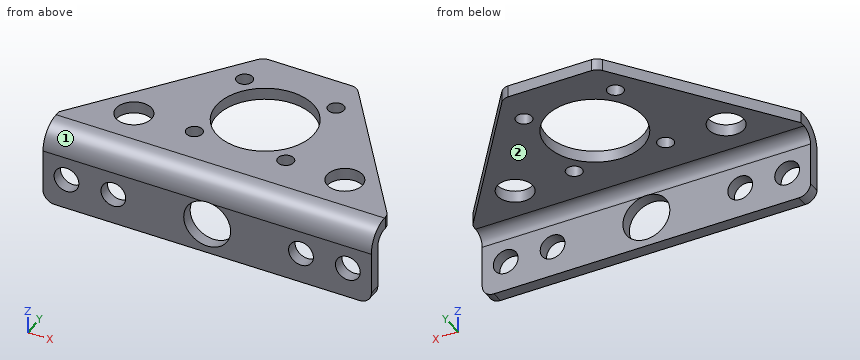
from build123d import *

# Parameters (mm, degrees)
BOSS_EXTRUDE1_DEPTH = 44.45
SKETCH2_OUTSIDE_W   = 111.802
SKETCH2_OUTSIDE_H   = 43.857
SKETCH2_OUTSIDE_R   = 3.3528
SKETCH2_OUTSIDE_R_2 = 6.35
CUT_EXTRUDE3_DEPTH  = 51.8
SKETCH3_OUTSIDE_W   = 111.802
SKETCH3_OUTSIDE_H   = 73.702
SKETCH3_OUTSIDE_R   = 2.1463
SKETCH3_OUTSIDE_R_2 = 13.0556
SKETCH3_OUTSIDE_R_3 = 4.7625
SKETCH3_OUTSIDE_R_4 = 4.743651166
CUT_EXTRUDE4_DEPTH  = 21.948744152


with BuildPart() as part:
    # Sketch1 → Boss-Extrude1 (new body, symmetric)
    with BuildSketch(Plane.ZY):
        with BuildLine():
            Line((-20.955, -28.575), (-6.5, -28.575))
            ThreePointArc((-6.5, -28.575), (-1.903805922, -26.671194078), (0, -22.075))
            Line((0, -22.075), (0, 22.225))
            Line((0, 22.225), (-3.175, 22.225))
            Line((-3.175, 22.225), (-3.175, -22.15))
            ThreePointArc((-3.175, -22.15), (-4.126902961, -24.448097039), (-6.425, -25.4))
            Line((-6.425, -25.4), (-20.955, -25.4))
            Line((-20.955, -25.4), (-20.955, -28.575))
        make_face()
    extrude(amount=BOSS_EXTRUDE1_DEPTH, both=True)

    # Sketch2 outside → Cut-Extrude3 (cut, through all)
    with BuildSketch(Plane.XZ.offset(28.575)):
        with Locations((0, -10.4775)):
            Rectangle(SKETCH2_OUTSIDE_W, SKETCH2_OUTSIDE_H)
        with BuildLine():
            Line((-41.280304188, -20.948744152), (41.275, -20.948744152))
            ThreePointArc((41.275, -20.948744152), (43.52006403, -20.018808183), (44.45, -17.773744152))
            Line((44.45, -17.773744152), (44.45, 4.535349672))
            Line((44.45, 4.535349672), (-44.455304188, 4.535349672))
            Line((-44.455304188, 4.535349672), (-44.455304188, -17.773744152))
            ThreePointArc((-44.455304188, -17.773744152), (-43.525368218, -20.018808183), (-41.280304188, -20.948744152))
        make_face(mode=Mode.SUBTRACT)
        with Locations((-38.1, -12.7)):
            Circle(SKETCH2_OUTSIDE_R)
        with Locations((-25.4, -12.7)):
            Circle(SKETCH2_OUTSIDE_R)
        with Locations((0, -12.7)):
            Circle(SKETCH2_OUTSIDE_R_2)
        with Locations((25.4, -12.7)):
            Circle(SKETCH2_OUTSIDE_R)
        with Locations((38.1, -12.7)):
            Circle(SKETCH2_OUTSIDE_R)
    extrude(amount=-CUT_EXTRUDE3_DEPTH, mode=Mode.SUBTRACT)

    # Sketch3 outside → Cut-Extrude4 (cut, through all)
    with BuildSketch(Plane.XY):
        with Locations((0, -3.175)):
            Rectangle(SKETCH3_OUTSIDE_W, SKETCH3_OUTSIDE_H)
        with BuildLine():
            Line((-13.653876698, 20.947210396), (-44.450826739, -20.631729198))
            Line((-44.450826739, -20.631729198), (-44.450826739, -28.575))
            Line((-44.450826739, -28.575), (44.45, -28.575))
            Line((44.45, -28.575), (44.45, -21.674369393))
            ThreePointArc((44.45, -21.674369393), (44.29004015, -20.679302615), (43.826278492, -19.784500865))
            Line((43.826278492, -19.784500865), (13.654037866, 20.947321174))
            ThreePointArc((13.654037866, 20.947321174), (12.531096243, 21.893026448), (11.102759374, 22.232452646))
            Line((11.102759374, 22.232452646), (-11.10251615, 22.232452646))
            ThreePointArc((-11.10251615, 22.232452646), (-12.530914579, 21.892995438), (-13.653876698, 20.947210396))
        make_face(mode=Mode.SUBTRACT)
        with Locations((-12.374792935, 12.374792935)):
            Circle(SKETCH3_OUTSIDE_R)
        with Locations((12.374792935, 12.374792935)):
            Circle(SKETCH3_OUTSIDE_R)
        Circle(SKETCH3_OUTSIDE_R_2)
        with Locations((-28.575, -12.7)):
            Circle(SKETCH3_OUTSIDE_R_3)
        with Locations((-12.374792935, -12.374792935)):
            Circle(SKETCH3_OUTSIDE_R)
        with Locations((12.374792935, -12.374792935)):
            Circle(SKETCH3_OUTSIDE_R)
        with Locations((28.564780042, -12.715837646)):
            Circle(SKETCH3_OUTSIDE_R_4)
    extrude(amount=-CUT_EXTRUDE4_DEPTH, mode=Mode.SUBTRACT)


solid = part.part
Check sheet for the modelled part. Datum: model origin and axes. Units: mm. Face numbers are marked on the shaded views. A direction names the side the tool comes from. Give positions to 0.01 mm unless a question says otherwise; leave off trailing zeros. Order: outer loops, then holes, each group sorted by start corner. A loop starts at its lowest first (then second) coordinate and runs counter-clockwise, first axis right, second up. Notation, with made-up numbers: M 9.25,-37.5 L 55.25,-37.5 A32 ccw 55.25,-7.5 Z; hole C 65,21.25 d6. An arc over 180 degrees is marked long. Answer as CSV lines item,"result". Start each with the question number.
Item 1: Cross-section at C-C on x = 38.1. Enter the section's corners in (y, z) (3 decimals).
Item 2: Cross-section at D-D on y = -2. Enter the section's corners in (x, z) (1 decimal).
Item 3: Cross-section at B-B on x = -25. Enter the section's corners in (y, z) (3 decimals).
Item 4: Gauge pin test, flat ends, axial feed: P1, Ø5, axis at x = 12.37, y = 12.37, coming from the -Z side (3 decimals); P2, Ø23.5, axis at x = 0, y = 0, coming from the -Z side; P3, Ø4, axis at y = 7, z = -4.5, coming from the -X side; P4, Ø12, axis at x = 13.5, z = -15.5, coming from the +Y side. Record the tip position at first contact, or that the pin passes through.
Item 5: Cross-section at A-A on z = -12.7. Enter the section's corners in (x, y) (3 decimals).
Item 6: Thickness scan on line 1 (Z direction, x = 31.5, y = -6.5) (3 decimals); line 2 (Y direction, x = 7, z = -7.5) (3 decimals); line 3 (Y direction, x = 11.5, z = -3). Record the ranges inside material, lowest first. Write a range as [from, to].
Item 7: Tool access check on the marked faces 1 and 2. Record the directions out of +Z, -Z, +X, -X, +Y, -Y that give a thin tool (end or side, any length) a straight path to the whole face; none if there is none.
Established:
1,outline,"M -28.575,-20.949 L -25.4,-20.949 L -25.4,-16.053 L -28.575,-16.053 Z; M -28.575,-9.347 L -25.4,-9.347 L -25.4,-6.425 A3.25 cw -22.15,-3.175 L -12.054,-3.175 L -12.054,0 L -22.075,0 A6.5 ccw -28.575,-6.5 Z"
2,outline,"M -30.7,-3.2 L -12.9,-3.2 L -12.9,0 L -30.7,0 Z; M 12.9,-3.2 L 30.7,-3.2 L 30.7,0 L 12.9,0 Z"
3,outline,"M -28.575,-20.949 L -25.4,-20.949 L -25.4,-16.029 L -28.575,-16.029 Z; M -28.575,-9.371 L -25.4,-9.371 L -25.4,-6.425 A3.25 cw -22.15,-3.175 L -15.847,-3.175 L -15.847,0 L -22.075,0 A6.5 ccw -28.575,-6.5 Z; M -9.553,-3.175 L 5.629,-3.175 L 5.629,0 L -9.553,0 Z"
4,P1,"stops at z = -3.175"
4,P2,"passes through"
4,P3,"stops at x = -25.09"
4,P4,"stops at y = -25.4"
5,outline,"M -44.45,-28.575 L -41.453,-28.575 L -41.453,-25.4 L -44.45,-25.4 Z; M -34.747,-28.575 L -28.753,-28.575 L -28.753,-25.4 L -34.747,-25.4 Z; M -22.047,-28.575 L -6.35,-28.575 L -6.35,-25.4 L -22.047,-25.4 Z; M 6.35,-28.575 L 22.047,-28.575 L 22.047,-25.4 L 6.35,-25.4 Z; M 28.753,-28.575 L 34.747,-28.575 L 34.747,-25.4 L 28.753,-25.4 Z; M 41.453,-28.575 L 44.45,-28.575 L 44.45,-25.4 L 41.453,-25.4 Z"
6,line 1,"z = [-3.175, 0]"
6,line 2,"y = [-28.575, -25.4]"
6,line 3,"y = [-27.55, -14.33], [-10.41, -6.18], [6.18, 10.41], [14.33, 22.21]"
7,face 1,"+Z, +X, -X, -Y"
7,face 2,"-Z, +X, -X, +Y"
